Could you check a few things on this model? Use its own coordinates, in mm. A direction names the side the tool comes from. Coordinates: 2 decimals unless noted, no trailing zeros. Order: outer loops, then holes, each group sorted by start corner. A loop starts at its lowest first (then second) coordinate and runs counter-clockwise, first axis right, second up. Notation, with made-up numbers: (48, 34.25) - (80, 34.25) arc R30 ccw to (80, 61.25) - close; hole circle Ø8 at (19.5, -21.5). An arc over 180 degrees is marked (long way). Answer as a JSON object with one key per item and string values. Group by question number.
(1) Imagine slicing it at A-A, the plane x = -31. Write out the boundary of the cut face in (y, z) (3 decimals).
(2) We'd pull the mould along Y, two halves only. Please class faces 3 (the flat face through (12, -3, 3.175)), 4 (the cylindrical face through (-56.99, 140.35, 1.57)), 5 (the cylindrical face through (-57.15, -140.51, 1.57)): pulls with the +Y half, pulls with the -Y half, needs draft (parallel to the pull), parting line crosses it, or undercut.
(3) Which directions (+Z, -Z, +X, -X, +Y, -Y) give clear straight access to the entire face, cutting with the end or side of a thin tool? Please do faces 1 (the flat face through (12, -3, 0)), 2 (the cylindrical face through (-13.01, -134.65, 1.57)).
(4) Please list where these lines run through material, in increasing order: probe 1 along X at (y, z) = (237.5, 1.9); probe 2 along Y at (x, z) = (-47.5, 2); probe 3 along Y at (x, z) = (-23.5, 2.8).
(5) Will these pins go through, and if not, where does the flat tip stop? P1, Ø5, axis at x = -47.5, y = -237.5, coming from the -Z side; P2, Ø1, axis at y = 46.5, z = 1, coming from the -X side; P3, Ø9, axis at x = -47.5, y = 237.5, coming from the -Z side.
(6) Imagine slicing it at B-B, the plane z = 0.8. Write out the boundary of the cut face in (x, y), and give its area (3 significant figures).
(7) Imagine slicing it at C-C, the plane y = 109.5. Write out the boundary of the cut face in (x, z) (3 decimals), and give its area (3 significant figures).
from build123d import *

# Parameters (mm, degrees)
SKETCH1_W           = 500
SKETCH1_H           = 120
SKETCH1_R           = 2.8
BOSS_EXTRUDE1_DEPTH = 3.175
SKETCH2_W           = 50
SKETCH2_H           = 275
CUT_EXTRUDE1_DEPTH  = 258.11880644
FILLET1_R           = 10
SKETCH3_W           = 120
SKETCH3_H           = 5
CUT_EXTRUDE2_DEPTH  = 258.11880644


with BuildPart() as part:
    # Sketch1 → Boss-Extrude1 (new body)
    with BuildSketch(Plane(origin=(0, 0, 0), x_dir=(0, 1, 0), z_dir=(0, 0, 1))):
        Rectangle(SKETCH1_W, SKETCH1_H)
        with Locations(Location((-237.5, 47.5, 0), (0, 0, 270))):
            Circle(SKETCH1_R, mode=Mode.SUBTRACT)
        with Locations(Location((-237.5, -47.5, 0), (0, 0, 270))):
            Circle(SKETCH1_R, mode=Mode.SUBTRACT)
        with Locations(Location((237.5, 47.5, 0), (0, 0, 270))):
            Circle(SKETCH1_R, mode=Mode.SUBTRACT)
        with Locations(Location((237.5, -47.5, 0), (0, 0, 270))):
            Circle(SKETCH1_R, mode=Mode.SUBTRACT)
    extrude(amount=BOSS_EXTRUDE1_DEPTH)

    # Sketch2 → Cut-Extrude1 (cut, through all)
    with BuildSketch(Plane.XY.offset(3.175)):
        with Locations((-35, 0)):
            Rectangle(SKETCH2_W, SKETCH2_H)
    extrude(amount=-CUT_EXTRUDE1_DEPTH, mode=Mode.SUBTRACT)

    # Fillet1
    fillet1_edges = [part.edges().sort_by_distance(p)[0] for p in [
        (-60, -137.5, 1.5875),
        (-60, 137.5, 1.5875),
        (-10, 137.5, 1.5875),
        (-10, -137.5, 1.5875),
    ]]
    fillet(fillet1_edges, radius=FILLET1_R)

    # Sketch3 → Cut-Extrude2 (cut, through all)
    with BuildSketch(Plane.XY.offset(3.175)):
        with Locations((0, 247.5)):
            Rectangle(SKETCH3_W, SKETCH3_H)
        with Locations((0, -247.5)):
            Rectangle(SKETCH3_W, SKETCH3_H)
    extrude(amount=-CUT_EXTRUDE2_DEPTH, mode=Mode.SUBTRACT)


solid = part.part
Result set:
{
 "1": {"outline": "(-245, 0) - (-137.5, 0) - (-137.5, 3.175) - (-245, 3.175) - close; (137.5, 0) - (245, 0) - (245, 3.175) - (137.5, 3.175) - close"},
 "2": {"face 3": "needs draft", "face 4": "undercut", "face 5": "undercut"},
 "3": {"face 1": "-Z, +X, -X, +Y, -Y", "face 2": "+Z, -Z, -X"},
 "4": {"probe 1": "x = -60 to -50.3, -44.7 to 44.7, 50.3 to 60", "probe 2": "y = -245 to -240.3, -234.7 to -137.5, 137.5 to 234.7, 240.3 to 245", "probe 3": "y = -245 to -137.5, 137.5 to 245"},
 "5": {"P1": "passes through", "P2": "stops at x = -10", "P3": "stops at z = 0"},
 "6": {"outline": "(-60, -245) - (60, -245) - (60, 245) - (-60, 245) - (-60, 147.5) arc R10 ccw to (-50, 137.5) - (-20, 137.5) arc R10 cw to (-10, 127.5) - (-10, -127.5) arc R10 cw to (-20, -137.5) - (-50, -137.5) arc R10 ccw to (-60, -147.5) - close; hole circle Ø5.6 at (-47.5, -237.5); hole circle Ø5.6 at (-47.5, 237.5); hole circle Ø5.6 at (47.5, -237.5); hole circle Ø5.6 at (47.5, 237.5)", "area": "45,000 mm^2"},
 "7": {"outline": "(-10, 0) - (60, 0) - (60, 3.175) - (-10, 3.175) - close", "area": "222 mm^2"}
}
